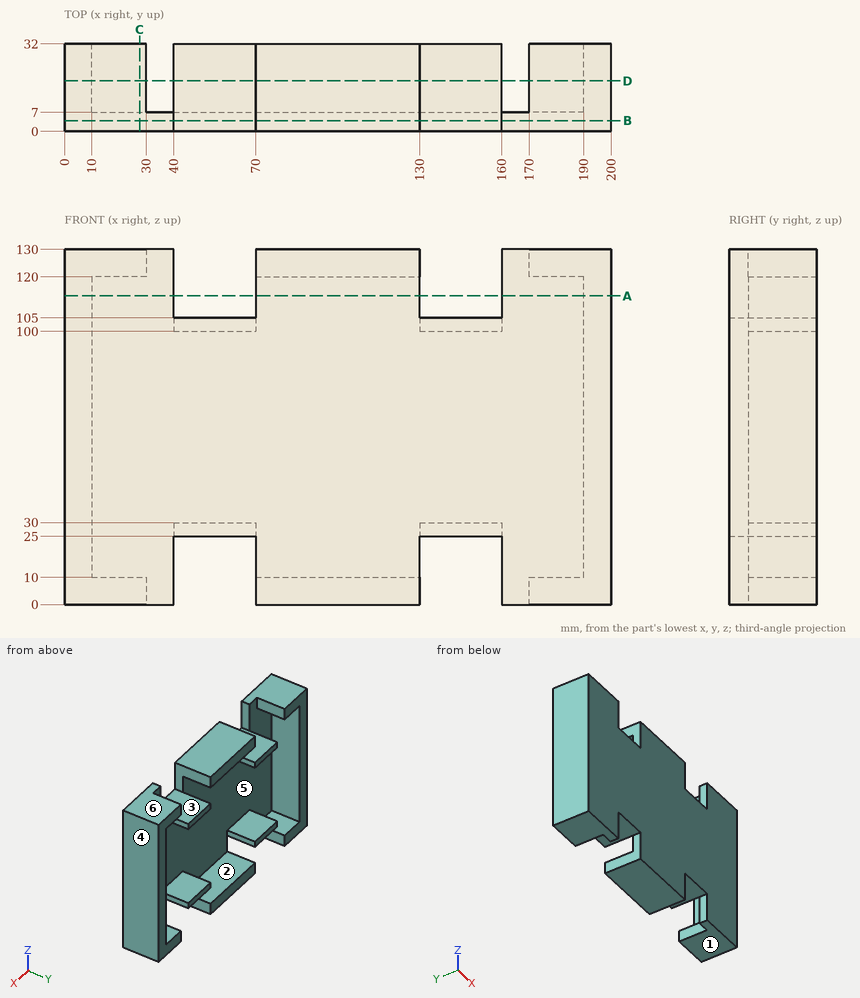
The figure shows three views and two pictorial views of one solid part (mm, origin at its lowest corner). Answer the questions. A direction names the side the tool comes from. Give positions to 0.01 mm unless a question says otherwise; leave off trailing zeros. Order: outer loops, then holes, each group sorted by start corner. A loop starts at its lowest first (then second) coordinate and runs counter-clockwise, first axis right, second up. Notation, with made-up numbers: (-8, -31.5) -> (16, -31.5) arc R29 ccw to (16, -1.5) -> close; hole circle Ø9 at (19.25, 14.5). An arc over 180 degrees is marked (long way). Answer as CSV lines item,"result". Start each with the question number.
Q1. Determine the mould class of the marked faces 4, 5 and 6 for opening direction Z: pulls with the +Z half, pulls with the -Z half, needs draft (parallel to the pull), parting line crosses it, or undercut.
Q2. Given pin 1 (2.5 mm diameter, centred on y = 18.5, z = 27, fed in from -X); pin 2 (3 mm diameter, centred on x = 59, y = 6, fed in from -Z); pin 3 (3 mm diameter, centred on x = 164.5, z = 113.5, fed in from +Y), each flat-ended and moving along its own axis, determine where each tip first touches the part or whether it passes through.
Q3. A cutting plane is placed at C-C (x = 27.5). Determine the outline of the cut face in (y, z).
Q4. Find the intervals of material crossed by L1, parallel to X at y = 5, z = 21.5; L2, parallel to X at y = 9, z = 102.5; L3, parallel to Z at x = 174.5, y = 12, in increasing order.
Q5. A cutting plane is placed at B-B (y = 4). Determine the outline of the cut face in (x, z).
Q6. Which of the six approach directions +Z, -Z, +X, -X, +Y, -Y give full straight-line access (tool end or side, diameter ignored) to the marked faces 1, 2 and 3?
Q7. A cutting plane is placed at D-D (y = 18.5). Count the separate pieces of the cut face and the enclosed holes in it, then the cut area to 3 significant figures.
Q8. A cutting plane is placed at A-A (z = 113). Determine the outline of the cut face in (x, y).
Results found:
1,face 4,"needs draft"
1,face 5,"undercut"
1,face 6,"pulls with the +Z half"
2,pin 1,"x = 0"
2,pin 2,"z = 25"
2,pin 3,"y = 7"
3,outline,"(0, 0) -> (32, 0) -> (32, 10) -> (7, 10) -> (7, 120) -> (32, 120) -> (32, 130) -> (0, 130) -> close"
4,L1,"0 to 40, 70 to 130, 160 to 200"
4,L2,"0 to 10, 40 to 70, 130 to 160, 190 to 200"
4,L3,"0 to 10, 120 to 130"
5,outline,"(0, 0) -> (40, 0) -> (40, 25) -> (70, 25) -> (70, 0) -> (130, 0) -> (130, 25) -> (160, 25) -> (160, 0) -> (200, 0) -> (200, 130) -> (160, 130) -> (160, 105) -> (130, 105) -> (130, 130) -> (70, 130) -> (70, 105) -> (40, 105) -> (40, 130) -> (0, 130) -> close"
6,face 1,"-Z, +X, -X, +Y, -Y"
6,face 2,"+Y"
6,face 3,"+Z, +Y, -Y"
7,separate pieces,"8"
7,enclosed holes,"0"
7,area,"5,200 mm2"
8,outline,"(0, 0) -> (40, 0) -> (40, 7) -> (10, 7) -> (10, 32) -> (0, 32) -> close; (70, 0) -> (130, 0) -> (130, 7) -> (70, 7) -> close; (160, 0) -> (200, 0) -> (200, 32) -> (190, 32) -> (190, 7) -> (160, 7) -> close"
